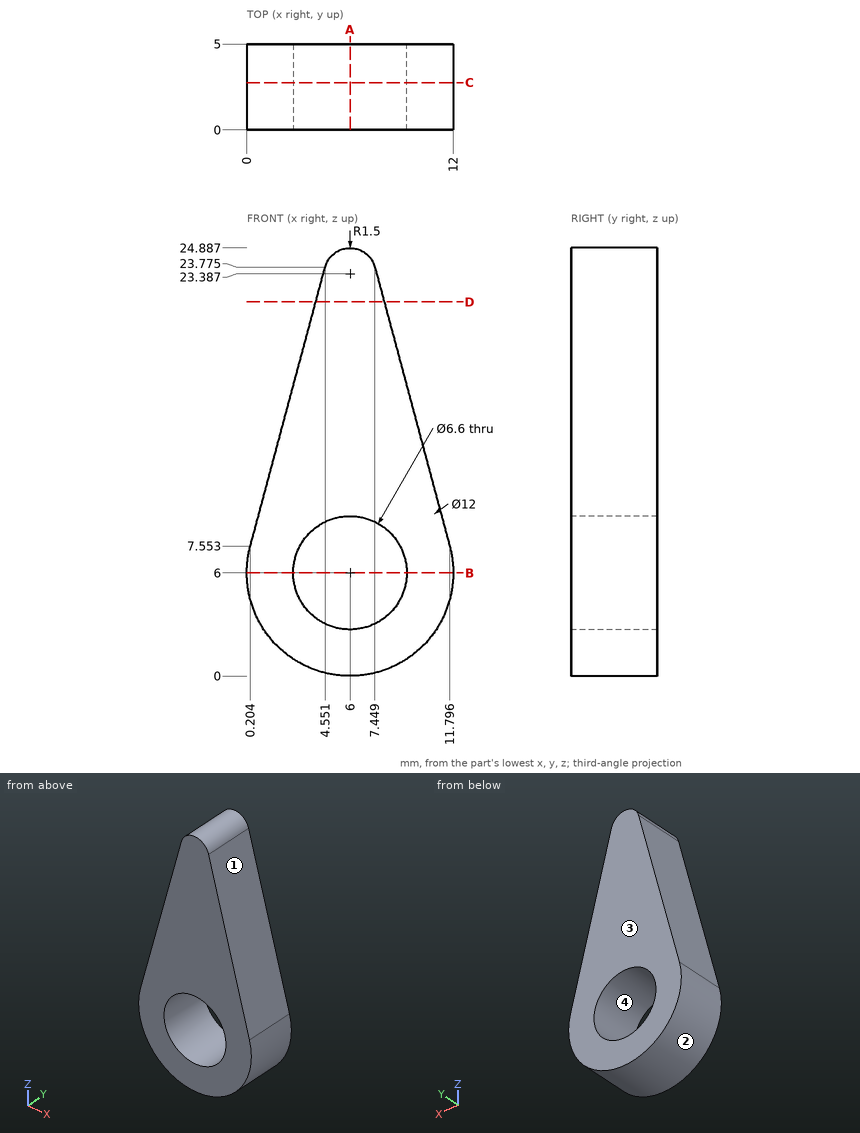
Input: dimensioned drawing with shaded views. Units: mm. Origin: part minimum x, y, z. Give positions to 0.01 mm unless a question says otherwise; leave off trailing zeros. Write each loop counter-clockwise with the first axis right and the second up, starting at its lowest first coordinate (ties: lowest second). Pieces come first, ordered by that corner, then holes. Notation, with made-up numbers: (7.25, 51) -> (37.25, 51) arc R22 ccw to (37.25, 68) -> close; hole circle Ø2 at (-11.75, 21). An arc over 180 degrees is marked (long way). Return JSON: item names as keys, results as strings. Group by question number.
1. Section A-A, the plane x = 6. Output: boundary loops of the cut face in (y, z).
2. Section C-C, the plane y = 2.75. Output: boundary loops of the cut face in (x, z) (1 decimal).
3. Section B-B, the plane z = 6. Output: boundary loops of the cut face in (x, y), then the cut area to 3 significant figures.
4. Material intervals for line 1 (X direction, y = 2.55, z = 6); line 2 (Z direction, x = 6, y = 3.35); line 3 (Z direction, x = 6.5, y = 1.6), sorted ascending. Write a range as from..to.
5. Pin query (flat end, axial travel): pin 1 Ø1 at (y, z) = (4.5, 15) entering from -X. Return the tip coordinate at first contact, or that it passes through.
6. Section D-D, the plane z = 21.75. Output: boundary loops of the cut face in (x, y).
7. Mould query, pull axis X, two halves, no side actions, for the marked faces 1, 2, 3 and 4. Classes: +X half, -X half, draft (parallel to the pull), parting line (faces both ways), or undercut.
Determined:
{
 "1": {"outline": "(0, 0) -> (5, 0) -> (5, 2.7) -> (0, 2.7) -> close; (0, 9.3) -> (5, 9.3) -> (5, 24.89) -> (0, 24.89) -> close"},
 "2": {"outline": "(0.2, 7.6) arc R6 ccw (long way) to (11.8, 7.6) -> (7.4, 23.8) arc R1.5 ccw to (4.6, 23.8) -> close; hole circle Ø6.6 at (6, 6)"},
 "3": {"outline": "(0, 0) -> (2.7, 0) -> (2.7, 5) -> (0, 5) -> close; (9.3, 0) -> (12, 0) -> (12, 5) -> (9.3, 5) -> close", "area": "27.0 mm2"},
 "4": {"line 1": "x = 0..2.7, 9.3..12", "line 2": "z = 0..2.7, 9.3..24.89", "line 3": "z = 0.02..2.74, 9.26..24.8"},
 "5": {"pin 1": "stops at x = 2.07"},
 "6": {"outline": "(4.01, 0) -> (7.99, 0) -> (7.99, 5) -> (4.01, 5) -> close"},
 "7": {"face 1": "+X half", "face 2": "parting line", "face 3": "draft", "face 4": "undercut"}
}
